Design review of the part shown in the three views and the two pictorial views. Dimensions are in mm from the part's minimum x, y and z. A direction names the side the tool comes from. Give positions to 0.01 mm unless a question says otherwise; leave off trailing zeros. Write each loop counter-clockwise with the first axis right and the second up, starting at its lowest first coordinate (ties: lowest second). Pieces come first, ordered by that corner, then holes. Notation, with made-up numbers: M 24,73 L 67,73 A23 ccw 67,99 Z; hole C 71,17.25 d10. An arc over 180 degrees is marked long. Use one line per item in the form item = value. Start each with the question number.
Q1. Consider section C-C on z = 1.5. Write out the cut boundary in (x, y).
Q2. Clearance check with flat-ended pins moving along their axes: pin 1 Ø2 at (y, z) = (2, 3) entering from +X; pin 2 Ø2 at (y, z) = (6, 3) entering from -X. State where each tip first meets the part, or that it passes through.
Q3. Tool access review of the marked faces 4, 5 and 6: name each direction out of +Z, -Z, +X, -X, +Y, -Y from which nothing blocks a thin tool from reaching the whole face with its end or side.
Q4. Consider section A-A on z = 3.5. Write out the cut boundary in (x, y), and give its area (4 significant figures).
Q5. Consider section D-D on y = 2.5. Write out the cut boundary in (x, z).
Q6. Mouldability with a two-part tool opening along Z and no side actions: class the marked faces 1, 2 and 3 as released by +Z, released by -Z, zero draft, split by the parting line, or undercut.
Q7. Consider section B-B on x = 5. Write out the cut boundary in (y, z), and give its area (3 significant figures).
Q8. For probe 1 along Z at (x, y) = (5, 1.45); probe 2 along X at (y, z) = (1.5, 5); probe 3 along X at (y, z) = (6.75, 4), list the stretches that pass through material, from the lowest coordinate up. Write a range as [from, to].
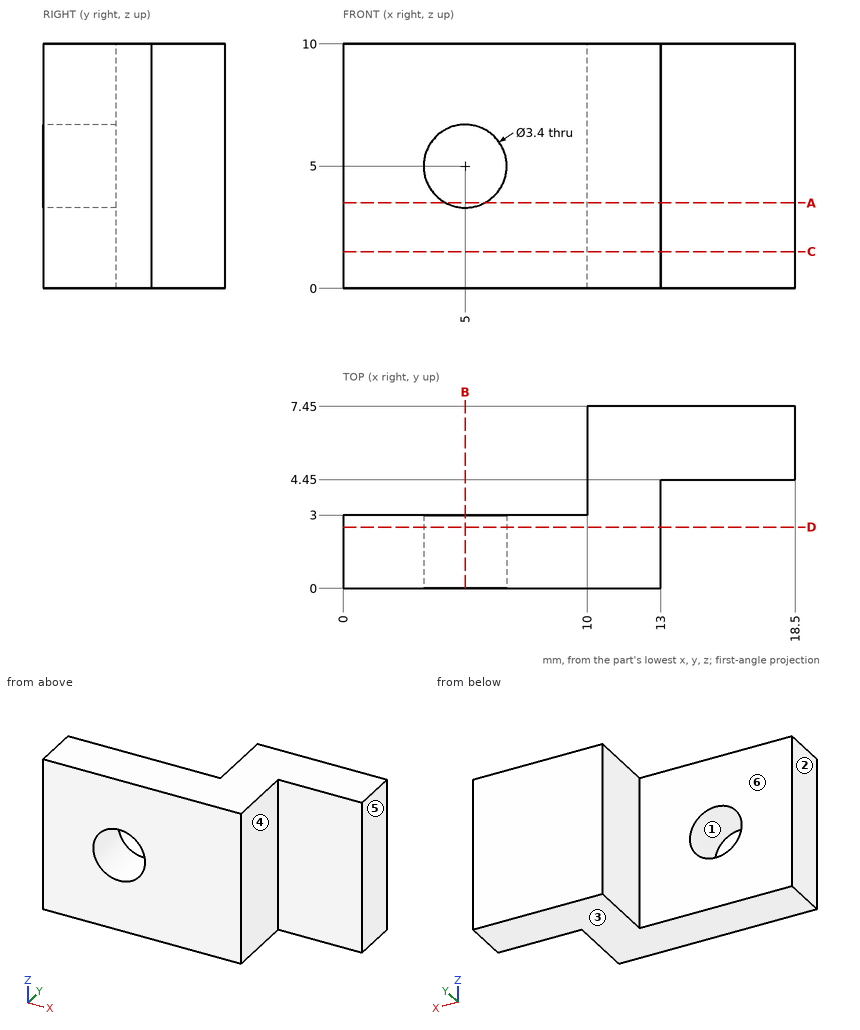
Working result:
q1.outline = M 0,0 L 13,0 L 13,4.45 L 18.5,4.45 L 18.5,7.45 L 10,7.45 L 10,3 L 0,3 Z
q2.pin_1 = 13
q2.pin_2 = 10
q3.face_4 = +Z, -Z, +X, -Y
q3.face_5 = +Z, -Z, +X, +Y, -Y
q3.face_6 = +Z, -Z, -X, +Y
q4.outline = M 0,0 L 4.2,0 L 4.2,3 L 0,3 Z; M 5.8,0 L 13,0 L 13,4.45 L 18.5,4.45 L 18.5,7.45 L 10,7.45 L 10,3 L 5.8,3 Z
q4.area = 64.05 mm²
q5.outline = M 0,0 L 13,0 L 13,10 L 0,10 Z; hole C 5,5 d3.4
q6.face_1 = undercut
q6.face_2 = zero draft
q6.face_3 = released by -Z
q7.outline = M 0,0 L 3,0 L 3,3.3 L 0,3.3 Z; M 0,6.7 L 3,6.7 L 3,10 L 0,10 Z
q7.area = 19.8 mm²
q8.probe_1 = [0, 3.3], [6.7, 10]
q8.probe_2 = [0, 3.3], [6.7, 13]
q8.probe_3 = [10, 18.5]
